Geometry: final body of the model. Coordinates: model frame, mm. Coordinates: 2 decimals unless noted, no trailing zeros. Order: outer loops, then holes, each group sorted by start corner. A loop starts at its lowest first (then second) coordinate and runs counter-clockwise, first axis right, second up. Notation, with made-up numbers: (9, -33.5) -> (31, -33.5) arc R12 cw to (31, -28.5) -> close; hole circle Ø10 at (89.5, -21.5). An arc over 180 degrees is marked (long way). Use one line per item in the form item = value.
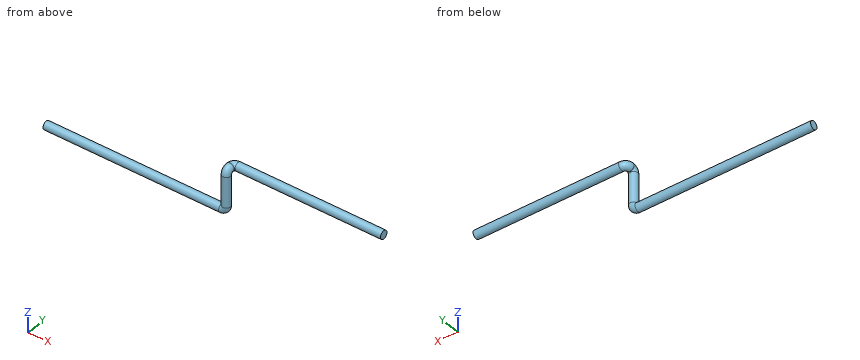
```python
from build123d import *

# Parameters (mm, degrees)
CROQUIS1_R = 13.7


with BuildPart() as part:
    # Barrer1: sweep along a curve in space
    with BuildLine() as barrer1_path:
        Line((0, 0, 0), (-485, 0, 0))
        ThreePointArc((-485, 0, 0), (-495.606601718, -4.393398282, 0), (-500, -15, 0))
        Line((-500, -15, 0), (-500, -16, 0))
        ThreePointArc((-500, -16, 0), (-500, -26.606601718, -4.393398282), (-500, -31, -15))
        Line((-500, -31, -15), (-500, -31, -115))
        ThreePointArc((-500, -31, -115), (-504.393398282, -31, -125.606601718), (-515, -31, -130))
        Line((-515, -31, -130), (-1100, -31, -130))
    # Croquis1 → Barrer1 (sweep)
    with BuildSketch(Plane(origin=(0, 0, 0), x_dir=(0, 0, -1), z_dir=(1, 0, 0))):
        Circle(CROQUIS1_R)
    sweep(path=barrer1_path.line)


solid = part.part
```
1) Contact query for flat-ended pins moving along their axis: P1, Ø8, axis at y = -36.5, z = -23, coming from the -X side; P2, Ø2, axis at y = -25, z = -113, coming from the -X side (3 decimals); P3, Ø12, axis at x = -541, y = -31.5, coming from the +Z side. Output: stop coordinate, or through.
Results found:
P1 = -513.62
P2 = -512.755
P3 = -116.3
2) Section A-A, the plane z = -65. Output: boundary loops of the cut face in (x, y).
Results found:
outline = circle Ø27.4 at (-500, -31)
3) Section B-B, the plane x = -329.5. Output: boundary loops of the cut face in (y, z), and give its area (3 significant figures).
Results found:
outline = circle Ø27.4 at (0, 0)
area = 590 mm2
4) Material intervals for probe 1 along X at (y, z) = (-17, 1); probe 2 along Z at (x, y) = (-797.5, -29); probe 3 along X at (y, z) = (-19, -2), sorted ascending. Write a range as from..to.
Results found:
probe_1 = -513.66..-486.34
probe_2 = -143.55..-116.45
probe_3 = -513.6..-486.4
